Input: dimensioned drawing with shaded views. Units: mm. Origin: part minimum x, y, z. A direction names the side the tool comes from. Round coordinates to 2 decimals unless told otherwise and drop trailing zeros. Loops run counter-clockwise (first coordinate to the right, second up) from the corner with the lowest first, then second, coordinate; pieces in that order, holes last.
1) Section D-D, the plane y = 89.5. Return loops of the section in (x, z) (1 decimal), and give its area (3 significant figures).
2) Access query for the marked faces 1, 2, 3 and 4. Directions: +Z, -Z, +X, -X, +Y, -Y. A direction counts if a zero-diameter tool reaches every point of the face in a straight line with its end or side. Return the directions, or none.
3) Section A-A, the plane z = 28.5. Return loops of the section in (x, y) (1 decimal), and give its area (3 significant figures).
4) Section B-B, the plane x = 103.5. Return loops of the section in (y, z), and give its area (3 significant figures).
5) First-contact query: pin 1 (1.4 mm diameter, centred on x = 2, y = 56.5, fed in from +Z); pin 2 (10 mm diameter, centred on y = 53, z = 33, fed in from -X); pin 3 (1.5 mm diameter, centred on y = 40.5, z = 19.5, fed in from +X). Flat tips, straight axial feed; report the tip coordinate or a pass-through.
6) Ray query, line 1 along X through (y, z) = (141.5, 50.5) (1 decimal); line 2 along Z through (x, y) = (94.5, 55.5); line 3 along X through (y, z) = (26, 9) (1 decimal). Return the intervals inside material, ascending.
7) Draft query along X for the marked faces 5, 6 and 7. Return one class per face: pulls with the +X half, pulls with the -X half, needs draft (parallel to the pull), parting line crosses it, or undercut.
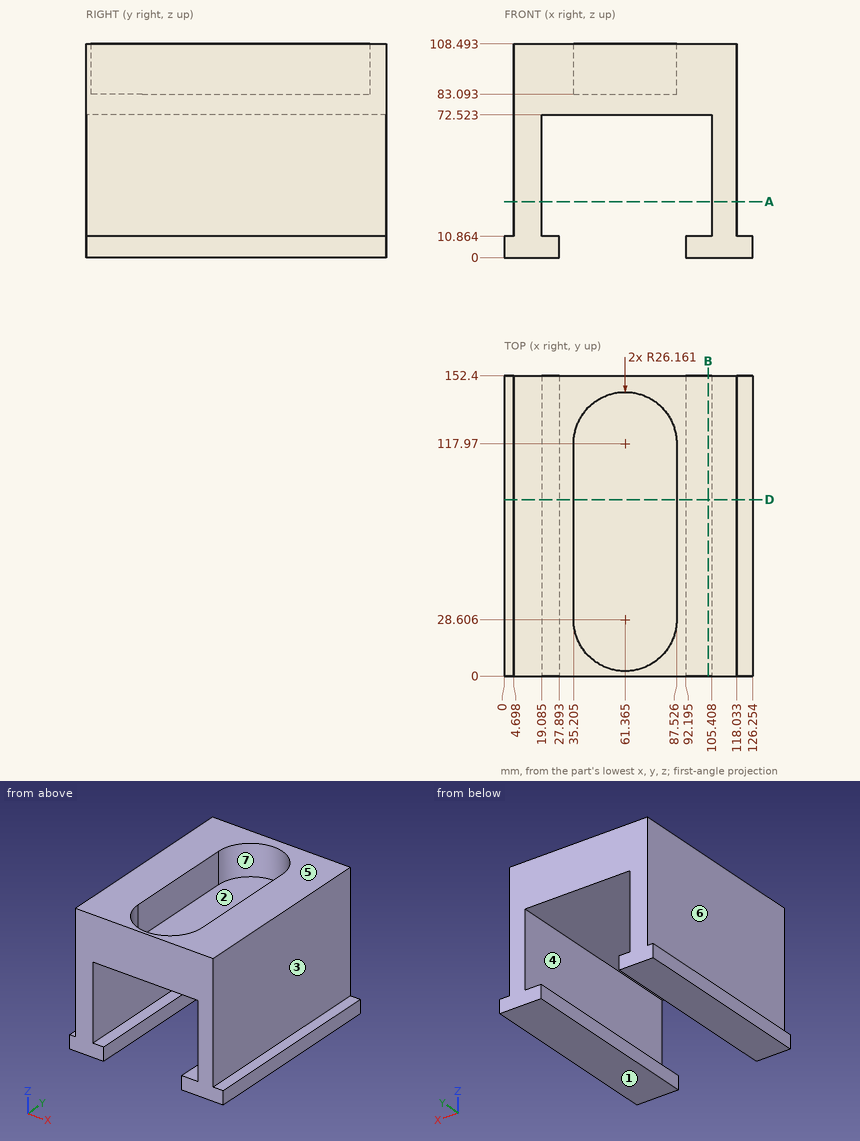
Final values:
1. outline: (0, 0) - (27.9, 0) - (27.9, 10.9) - (19.1, 10.9) - (19.1, 72.5) - (105.4, 72.5) - (105.4, 10.9) - (92.2, 10.9) - (92.2, 0) - (126.3, 0) - (126.3, 10.9) - (118, 10.9) - (118, 108.5) - (87.5, 108.5) - (87.5, 83.1) - (35.2, 83.1) - (35.2, 108.5) - (4.7, 108.5) - (4.7, 10.9) - (0, 10.9) - close
1. area: 5,090 mm2
2. face 1: -Z, +X, -X, +Y, -Y
2. face 2: +Z
2. face 3: +Z, +X, +Y, -Y
2. face 4: +Y, -Y
3. outline: (4.7, 0) - (19.1, 0) - (19.1, 152.4) - (4.7, 152.4) - close; (105.4, 0) - (118, 0) - (118, 152.4) - (105.4, 152.4) - close
3. area: 4,120 mm2
4. outline: (0, 0) - (152.4, 0) - (152.4, 10.86) - (0, 10.86) - close; (0, 72.52) - (152.4, 72.52) - (152.4, 108.49) - (0, 108.49) - close
4. area: 7,140 mm2
5. pin 1: stops at z = 10.86
5. pin 2: stops at x = 4.7
5. pin 3: stops at x = 118.03
6. line 1: x = 4.7 to 19.1, 105.4 to 118
6. line 2: z = 0 to 10.86, 72.52 to 108.49
6. line 3: x = 0 to 27.9, 92.2 to 126.3
7. face 5: needs draft
7. face 6: pulls with the -X half
7. face 7: undercut
